Autodesk Inventor part; units mm, degrees
ref_plane "YZ Plane" through (0, 0, 0) normal (1, 0, 0) x (0, 1, 0)
ref_plane "XZ Plane" through (0, 0, 0) normal (0, 1, 0) x (-1, 0, 0)
ref_plane "XY Plane" through (0, 0, 0) normal (0, 0, 1) x (1, 0, 0)
sketch "Эскиз1" plane through (0, 0, 0) normal (0, 0, 1) x (1, 0, 0)
  circle A0 centre (0, 0) radius 47.5
  dimension "d0" = 95
extrude "Выдавливание1" add sketch "Эскиз1" along normal blind 10
sketch "Эскиз2" plane through (0, 0, 10) normal (0, 0, 1) x (1, 0, 0)
  circle A0 centre (0, 0) radius 24
  dimension "d3" = 48
extrude "Выдавливание2" add sketch "Эскиз2" along normal blind 17
sketch "Эскиз4" plane through (0, 0, 10) normal (0, 0, 1) x (1, 0, 0)
  line L0 (0, 0) -> (34, 0)
  circle A0 centre (34, 0) radius 5
  circle A1 centre (0, 34) radius 5
  circle A2 centre (-34, 0) radius 5
  circle A3 centre (0, -34) radius 5
  dimension "d9" = 34
  dimension "d10" = 10
  dimension "d13" = 360
extrude "Выдавливание4" cut sketch "Эскиз4" against normal through all
sketch "Эскиз5" plane through (0, 0, 0) normal (0, 1, 0) x (-1, 0, 0)
  line L0 (0, 27) -> (0, 60)
  line L1 (0, 60) -> (20, 60)
  line L2 (20, 60) -> (20, 32.3071)
  line L3 (20, 32.3071) -> (19.0464, 31.3536)
  line L4 (18.9, 31) -> (18.9, 28)
  arc A0 (18.9, 28) -> (19.9, 27) centre (19.9, 28) ccw
  arc A1 (19.0464, 31.3536) -> (18.9, 31) centre (19.4, 31) ccw
  line L5 (0, 27) -> (19.9, 27)
  line L6 (24, 27) -> (-24, 27)
  line L7 (0, -12) -> (0, 72)
  point P0 (0, 0)
  dimension "d17" = 33
  dimension "d18" = 20
  dimension "d19" = 18.9
  dimension "d20" = 1
  dimension "d21" = 45
  dimension "d22" = 0.5
revolve "Вращение1" add sketch "Эскиз5" angle 360 about axis through (0, 0, -10) along (0, 0, 1)
chamfer "Фаска1" distance 1.6 angle 45 1 edges at (20, 0, 60)
thread "Резьба1"
sketch "Эскиз6" plane through (0, 0, 60) normal (0, 0, 1) x (1, 0, 0)
  circle A0 centre (0, 0) radius 12
  dimension "d30" = 24
sketch "Эскиз7" plane through (0, 0, 0) normal (0, 0, -1) x (-1, 0, 0)
  circle A0 centre (0, 0) radius 20
  dimension "d31" = 40
extrude "Выдавливание5" cut sketch "Эскиз7" against normal blind 20
extrude "Выдавливание6" cut sketch "Эскиз6" against normal through all
sketch "Эскиз8" plane through (0, 0, 0) normal (0, 1, 0) x (-1, 0, 0)
  circle A0 centre (0, 17) radius 6
  line L0 (0, -16.4988) -> (0, 98.9927)
  line L1 (47.5, 10) -> (-47.5, 10)
  point P0 (0, 0)
  dimension "d36" = 12
  dimension "d37" = 7
extrude "Выдавливание7" cut sketch "Эскиз8" along normal through all both and the other way through all
properties part number "РК3"
Geometry: final body of the model. Coordinates: model frame, mm. A direction names the side the tool comes from. Coordinates: 2 decimals unless noted, no trailing zeros. Write each loop counter-clockwise with the first axis right and the second up, starting at its lowest first coordinate (ties: lowest second). Pieces come first, ordered by that corner, then holes. Notation, with made-up numbers: (38.5, 54.5) - (70.5, 54.5) arc R21 cw to (70.5, 91.5) - close; hole circle Ø8 at (27.5, 64). An arc over 180 degrees is marked (long way). Return JSON: item names as keys, results as strings.
Item 1: Section query A-A (x = 31). Output: boundary loops of the cut face in (y, z), and give its area (3 significant figures).
Completed:
{"outline": "(-35.99, 0) - (-4, 0) - (-4, 10) - (-35.99, 10) - close; (4, 0) - (35.99, 0) - (35.99, 10) - (4, 10) - close", "area": "640 mm2"}
Item 2: Section query C-C (y = -2.5). Count the separate pieces of the cut face and the enclosed holes in it, and give its area (3 significant figures).
Completed:
{"separate pieces": "4", "enclosed holes": "0", "area": "1,150 mm2"}
Item 3: Line query: L1, parallel to Y at x = 0, z = 8; L2, parallel to Y at x = 4, z = 3.5; L3, parallel to Z at x = 28.5, y = -23.5. Output: solid intervals per line, ascending.
Completed:
{"L1": "y = -47.5 to -39, -29 to -20, 20 to 29, 39 to 47.5", "L2": "y = -47.33 to -37, -31 to -19.6, 19.6 to 31, 37 to 47.33", "L3": "z = 0 to 10"}
Item 4: Section query B-B (z = 17). Output: boundary loops of the cut face in (x, y).
Completed:
{"outline": "(-6, -23.24) - (-6, -19.08) arc R20 cw to (-6, 19.08) - (-6, 23.24) arc R24 ccw to start; (6, -23.24) arc R24 ccw to (6, 23.24) - (6, 19.08) arc R20 cw to (6, -19.08) - close"}
Item 5: Reachability of faces 1 (the face through (-2.601, -11.715, 40.28)), 2 (the face through (-18.475, -7.66, 9.86)), 3 (the face through (11.075, 21.292, 18.381)) from +Z, -Z, +X, -X, +Y, -Y: full face, straight path, thin tool, end or side. Return the list, or none.
Completed:
{"face 1": "+Z, -Z", "face 2": "-Z", "face 3": "+Z"}
Item 6: Pin query (flat end, axial travel): pin 1 Ø6 at (x, z) = (-34.5, 7) entering from -Y; pin 2 Ø8 at (x, y) = (0, 34) entering from +Z; pin 3 Ø5 at (y, z) = (-15.5, 10) entering from -X; pin 4 Ø10 at (y, z) = (19.5, 46.5) entering from -X (3 decimals). Return the tip coordinate at first contact, or that it passes through.
Completed:
{"pin 1": "stops at y = -35.55", "pin 2": "passes through", "pin 3": "stops at x = -45.69", "pin 4": "stops at x = -13.775"}
Item 7: Pull-direction query (X, two-part tool) for faces 4 (the face through (-18.027, 5.677, 29.479)), 5 (the face through (-4, 12, 60)), 6 (the face through (-1.08, -38.88, 5.07)); classes: +X half, -X half, draft (parallel to the pull), parting line (faces both ways), or undercut.
Completed:
{"face 4": "parting line", "face 5": "draft", "face 6": "undercut"}
